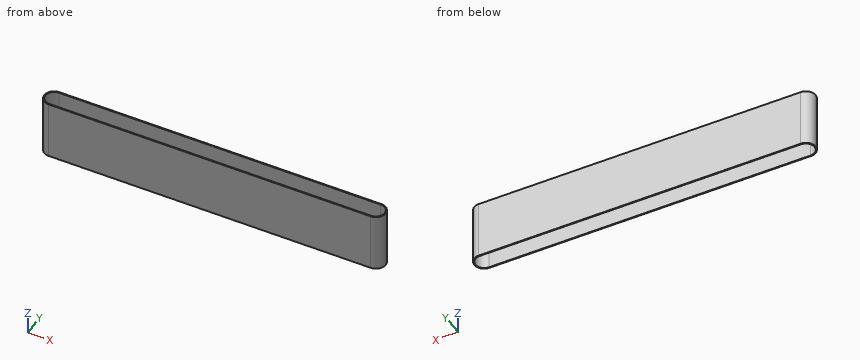
Autodesk Inventor part; units mm, degrees
ref_plane "YZ Plane" through (0, 0, 0) normal (1, 0, 0) x (0, 1, 0)
ref_plane "XZ Plane" through (0, 0, 0) normal (0, 1, 0) x (-1, 0, 0)
ref_plane "XY Plane" through (0, 0, 0) normal (0, 0, 1) x (1, 0, 0)
sketch "Boceto1" plane through (0, 0, 0) normal (0, 0, 1) x (1, 0, 0)
  arc A0 (275.236, 12.4594) -> (275.236, 45.4594) centre (275.2631, 28.9594) ccw
  line L0 (275.236, 12.4594) -> (-274.7368, 12.4594)
  arc A1 (-274.7368, 45.4594) -> (-274.7368, 12.4594) centre (-274.7368, 28.9594) ccw
  line L1 (-274.7368, 45.4594) -> (275.236, 45.4594)
  point P0 (0, 0)
  point P1 (0, 43.9853)
  point P2 (0, 13.9594)
  point P3 (290.2632, 28.9594)
  point P4 (-289.7368, 28.9594)
  dimension "d5" = 580
extrude "Extrusión1" add sketch "Boceto1" along normal blind 100
sketch "Boceto2" plane through (0, 0, 100) normal (0, 0, 1) x (1, 0, 0)
  line L0 (-274.4457, 43.9128) -> (274.9443, 43.9128)
  line L1 (275.236, 45.4594) -> (-274.7368, 45.4594)
  line L2 (274.9443, 13.9446) -> (-274.4457, 13.9446)
  line L3 (-274.7368, 12.4594) -> (275.236, 12.4594)
  arc A0 (-274.4457, 43.9128) -> (-274.4457, 13.9446) centre (-274.4457, 28.9287) ccw
  arc A1 (274.9443, 13.9446) -> (274.9443, 43.9128) centre (274.9443, 28.9287) ccw
  arc A2 (-274.7368, 45.4594) -> (-274.7368, 12.4594) centre (-274.7368, 28.9594) ccw
  point P0 (0, 0)
  dimension "d18" = 549.39
extrude "Extrusión2" cut sketch "Boceto2" against normal blind 100
properties part number "Banda" material "Caucho, Silicona"
Part model, mm, in its own coordinate system. Coordinates: 2 decimals unless noted, no trailing zeros. Loops run counter-clockwise (first coordinate to the right, second up) from the corner with the lowest first, then second, coordinate; pieces in that order, holes last. Notation, with made-up numbers: (-16.5, 11.25) -> (37.5, 11.25) arc R14 ccw to (37.5, 25.25) -> close; hole circle Ø9 at (47, -1). An arc over 180 degrees is marked (long way). Use a Markdown table: item, result. Add a question column.
Item 1: Flat gauge pins, fed straight in: P1, Ø6, axis at y = 33.5, z = 28, coming from the -X side; P2, Ø8, axis at y = 32, z = 65, coming from the +X side. Where does each tip first touch, or does it go through?
Item 2: Band-saw the part on B-B on y = 29. Write the cut outline in (x, z), plus the area to 3 significant figures.
Item 3: Band-saw the part on C-C on z = 82. Write the cut outline in (x, y), plus the area to 3 significant figures.
Item 4: Band-saw the part on A-A on x = 66. Write the cut outline in (y, z), plus the area to 3 significant figures.
Item 5: Probe probe 1 along Y at (x, z) = (27.5, 73.5); probe 2 along X at (y, z) = (29, 76); probe 3 along X at (y, z) = (27, 6). List the from-to ranges inside material, lowest first.
Geometry says:
| question | item | result |
|---|---|---|
| 1 | P1 | x = -291.16 |
| 1 | P2 | x = 291.76 |
| 2 | outline | (-291.24, 0) -> (-289.43, 0) -> (-289.43, 100) -> (-291.24, 100) -> close; (289.93, 0) -> (291.76, 0) -> (291.76, 100) -> (289.93, 100) -> close |
| 2 | area | 364 mm² |
| 3 | outline | (-274.74, 12.46) -> (275.24, 12.46) arc R16.5 ccw to (275.24, 45.46) -> (-274.74, 45.46) arc R16.5 ccw to start; hole (-274.45, 13.94) -> (274.94, 13.94) arc R14.98 ccw to (274.94, 43.91) -> (-274.45, 43.91) arc R14.98 ccw to start |
| 3 | area | 1,840 mm² |
| 4 | outline | (12.46, 0) -> (13.94, 0) -> (13.94, 100) -> (12.46, 100) -> close; (43.91, 0) -> (45.46, 0) -> (45.46, 100) -> (43.91, 100) -> close |
| 4 | area | 303 mm² |
| 5 | probe 1 | 12.46 to 13.94, 43.91 to 45.46 |
| 5 | probe 2 | -291.24 to -289.43, 289.93 to 291.76 |
| 5 | probe 3 | -291.12 to -289.31, 289.8 to 291.65 |
